CAD build for the part. Positions are in the model's coordinates, mm. Face numbers are marked on the shaded views. A direction names the side the tool comes from. Give positions to 0.01 mm unless a question says otherwise; leave off trailing zeros. Loops run counter-clockwise (first coordinate to the right, second up) from the corner with the lowest first, then second, coordinate; pieces in that order, holes last. Notation, with made-up numbers: (76.25, -11.75) - (85.25, -11.75) arc R5 ccw to (85.25, -2.75) - close; hole circle Ø10 at (9.5, 63.25). An arc over 180 degrees is marked (long way). Return JSON: item names as keys, results as strings.
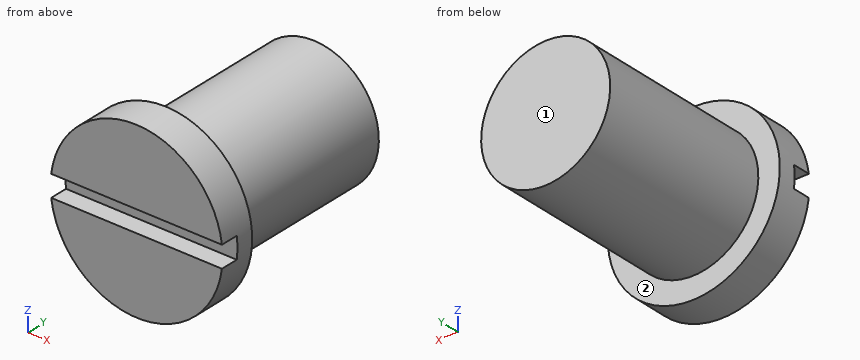
from build123d import *

# Parameters (mm, degrees)
ESQUISSE1_R             = 2.4
ESQUISSE1_R_2           = 1.8
BOSS_EXTRU_1_DEPTH      = 1
ESQUISSE2_R             = 1.8
BOSS_EXTRU_2_DEPTH      = 5
ENL_V_MAT_EXTRU_1_DEPTH = 0.5


with BuildPart() as part:
    # Esquisse1 → Boss.-Extru.1 (new body)
    with BuildSketch(Plane(origin=(0, 0, 0), x_dir=(1, 0, 0), z_dir=(0, 1, 0))):
        with Locations(Location((0, 0, 0), (0, 0, 270))):
            Circle(ESQUISSE1_R)
        Circle(ESQUISSE1_R_2, mode=Mode.SUBTRACT)
        Circle(ESQUISSE1_R_2)
    extrude(amount=BOSS_EXTRU_1_DEPTH)

    # Esquisse2 → Boss.-Extru.2 (add)
    with BuildSketch(Plane(origin=(0, 1, 0), x_dir=(1, 0, 0), z_dir=(0, 1, 0))):
        with Locations(Location((0, 0, 0), (0, 0, 270))):
            Circle(ESQUISSE2_R)
    extrude(amount=BOSS_EXTRU_2_DEPTH)

    # Esquisse3 → Enlèv. mat.-Extru.1 (cut)
    with BuildSketch(Plane.XZ):
        Polygon((2.4, 0), (2.4, -0.3), (-2.4, -0.3), (-2.4, 0), (-2.4, 0.297130131), (2.4, 0.297130131), align=None)
    extrude(amount=-ENL_V_MAT_EXTRU_1_DEPTH, mode=Mode.SUBTRACT)


solid = part.part
1. Drill centre lines: probe 1 along Y at (x, z) = (-1.25, 1.9); probe 2 along Z at (x, y) = (-0.05, 3); probe 3 along Z at (x, y) = (-0.25, 0.4). Where is each one in solid material? Low to high.
Values follow:
{"probe 1": "y = 0 to 1", "probe 2": "z = -1.8 to 1.8", "probe 3": "z = -2.39 to -0.3, 0.3 to 2.39"}
2. Cut at A-A, the plane x = 0. Write the cut outline in (y, z).
Values follow:
{"outline": "(0, -2.4) - (1, -2.4) - (1, -1.8) - (6, -1.8) - (6, 1.8) - (1, 1.8) - (1, 2.4) - (0, 2.4) - (0, 0.3) - (0.5, 0.3) - (0.5, -0.3) - (0, -0.3) - close"}
3. Cut at D-D, the plane x = 0.65. Write the cut outline in (y, z), plus the area to 3 significant figures.
Values follow:
{"outline": "(0, -2.31) - (1, -2.31) - (1, -1.68) - (6, -1.68) - (6, 1.68) - (1, 1.68) - (1, 2.31) - (0, 2.31) - (0, 0.3) - (0.5, 0.3) - (0.5, -0.3) - (0, -0.3) - close", "area": "21.1 mm²"}
4. Cut at C-C, the plane y = 0.75. Write the cut outline in (x, z), plus the area to 3 significant figures.
Values follow:
{"outline": "circle Ø4.8 at (0, 0)", "area": "18.1 mm²"}
5. Drop flat-ended pins along their axis: P1, Ø0.6, axis at x = 0.5, y = 0.5, coming from the +Z side; P2, Ø1, axis at y = 5, z = -0.5, coming from the +X side; P3, Ø1.5, axis at x = 1, y = 3, coming from the -Z side. Give the stop position or say it passes through.
Values follow:
{"P1": "stops at z = 2.39", "P2": "stops at x = 1.8", "P3": "stops at z = -1.78"}
6. Which spindle directions (+Z, -Z, +X, -X, +Y, -Y) get a long thin tool onto all of the face, cutting with end or side? Do the marked faces 1 and 2. Say none if no direction does.
Values follow:
{"face 1": "+Z, -Z, +X, -X, +Y", "face 2": "+Y"}
7. Cut at B-B, the plane z = 0. Write the cut outline in (x, y), plus the area to 3 significant figures.
Values follow:
{"outline": "(-2.4, 0.5) - (2.4, 0.5) - (2.4, 1) - (1.8, 1) - (1.8, 6) - (-1.8, 6) - (-1.8, 1) - (-2.4, 1) - close", "area": "20.4 mm²"}
